from build123d import *

# Parameters (mm, degrees)
SKETCH1_R                = 3
BOSS_EXTRUDE1_DEPTH      = 32.5
BOSS_EXTRUDE2_DEPTH      = 6.35
BOSS_EXTRUDE3_REACH      = 87.109
BOSS_EXTRUDE3_END_RADIUS = 7.62
BOSS_EXTRUDE3_START      = 18
SKETCH3_R                = 3.25
SKETCH4_R                = 6
BOSS_EXTRUDE4_DEPTH      = 18


with BuildPart() as part:
    # Sketch1 → Boss-Extrude1 (new, symmetric)
    with BuildSketch(Plane(origin=(0, 0, 0), x_dir=(1, 0, 0), z_dir=(0, 1, 0))):
        with Locations(Location((0, 0, 0), (0, 0, 270))):
            Circle(SKETCH1_R)
    extrude(amount=BOSS_EXTRUDE1_DEPTH, both=True)

    # Sketch2 → Boss-Extrude2 (add, symmetric)
    with BuildSketch(Plane.XY):
        with BuildLine():
            Line((-53.975, 20.32), (-53.975, 20.828))
            add(Edge.make_bspline(
                [(-53.975, 20.828), (-48.579084473, 22.104261863), (-42.739180184, 28.451304863), (-32.707581635, 36.217235943), (-19.445903171, 37.601432098), (-9.805142387, 34.528428283), (-4.615884318, 37.812838606)],
                knots=[0, 0, 0, 0, 0.290913355, 0.472280192, 0.684923774, 1, 1, 1, 1], degree=3))
            ThreePointArc((-4.615884318, 37.812838606), (7.434387163, 30.07838775), (-6.766850807, 28.24655453))
            ThreePointArc((-6.766850807, 28.24655453), (-8.671850807, 29.405444626), (-10.576850807, 28.24655453))
            add(Edge.make_bspline(
                [(-53.975, 20.32), (-46.121670197, 21.895048491), (-37.272795223, 34.142014089), (-20.262703733, 35.94817115), (-10.576850807, 28.24655453)],
                knots=[0, 0, 0, 0, 0.320306102, 1, 1, 1, 1], degree=3))
        make_face()
    extrude(amount=BOSS_EXTRUDE2_DEPTH, both=True)

    # Boss-Extrude3: up to this cylinder (the profile starts outside it)
    boss_extrude3_end = Plane(origin=(0, 31.75, 0), z_dir=(0, 0, -1)) * Cylinder(BOSS_EXTRUDE3_END_RADIUS, 190.458, mode=Mode.PRIVATE)
    # Sketch3 → Boss-Extrude3 (add, up to the surface)
    with BuildSketch(Plane(origin=(0, 0, 0), x_dir=(1, 0, 0), z_dir=(0, 1, 0)).offset(BOSS_EXTRUDE3_START), mode=Mode.PRIVATE) as boss_extrude3_sk1:
        with Locations(Location((0, 0, 0), (0, 0, 90))):
            Circle(SKETCH3_R)
    boss_extrude3_tool1 = extrude(boss_extrude3_sk1.sketch, amount=BOSS_EXTRUDE3_REACH, mode=Mode.PRIVATE) - boss_extrude3_end
    add(boss_extrude3_tool1.solids().sort_by_distance((0, 18, 0))[0])

    # Sketch4 → Boss-Extrude4 (add)
    with BuildSketch(Plane.XZ.offset(32.5)):
        with Locations(Location((0, 0, 0), (0, 0, 270))):
            Circle(SKETCH4_R)
    extrude(amount=-BOSS_EXTRUDE4_DEPTH)


solid = part.part
Source: CAD feature listing. Evaluate the final solid. Frame: model axes, mm. A direction names the side the tool comes from. Coordinates: 2 decimals unless noted, no trailing zeros. Order: outer loops, then holes, each group sorted by start corner. A loop starts at its lowest first (then second) coordinate and runs counter-clockwise, first axis right, second up. Notation, with made-up numbers: M -25.75,10 L -3.75,10 A22 ccw -3.75,32 Z; hole C -10,-18.75 d10. An arc over 180 degrees is marked long. Write each question's results on one line, items separated by ' | '. Start each with the question number.
1. Section B-B, the plane y = -11.5. Return the cut outline in (x, z).
2. Material intervals for L1, parallel to X at y = 31, z = -4.5; L2, parallel to X at y = 27, z = -5.5; L3, parallel to Y at x = -15, z = 0.75, sorted ascending.
3. Reachability of faces 4 (the face through (-3.222, 21.381, 0.423)), 5 (the face through (1.802, -23.626, -5.723)), 6 (the face through (0, -32.5, 0)) from +Z, -Z, +X, -X, +Y, -Y: full face, straight path, thin tool, end or side. Return the list, or none.
4. Draft query along Y for faces 1 (the face through (-8.639, 29.405, 0.089)), 2 (the face through (3, -14.5, -1)), 3 (the face through (-9, 31, -6.35)). Return one class per face: +Y half, -Y half, draft (parallel to the pull), parting line (faces both ways), or undercut.
5. Pin query (flat end, axial travel): pin 1 (4 mm diameter, centred on x = -47.5, z = 1, fed in from +Y); pin 2 (1.5 mm diameter, centred on y = 16, z = -1, fed in from +X); pin 3 (1 mm diameter, centred on y = -25, z = 3.5, fed in from -X). Return the tip coordinate at first contact, or that it passes through.
6. Section A-A, the plane x = 0. Return the cut outline in (y, z).
Solution:
1) outline: C 0,0 d6
2) L1: -39.27 to -35.98, -14.8 to 7.58 | L2: -43.8 to -41.6, -5.96 to 5.96 | L3: 31.1 to 36.06
3) face 4: none | face 5: -Y | face 6: +Z, -Z, +X, -X, -Y
4) face 1: -Y half | face 2: undercut | face 3: draft
5) pin 1: y = 25.51 | pin 2: x = 2.99 | pin 3: x = -5.2
6) outline: M -32.5,-6 L -14.5,-6 L -14.5,-3 L 18,-3 L 18,-3.25 L 24.13,-3.25 L 24.13,-6.35 L 39.37,-6.35 L 39.37,6.35 L 24.13,6.35 L 24.13,3.25 L 18,3.25 L 18,3 L -14.5,3 L -14.5,6 L -32.5,6 Z
